Autodesk Inventor part; units mm, degrees
ref_plane "YZ Plane" through (0, 0, 0) normal (1, 0, 0) x (0, 1, 0)
ref_plane "XZ Plane" through (0, 0, 0) normal (0, 1, 0) x (-1, 0, 0)
ref_plane "Arbeitsebene1" through (0, 0, -6) normal (0, 0, 1) x (1, 0, 0)
sketch "Skizze1" plane through (0, 0, -6) normal (0, 0, 1) x (1, 0, 0)
  circle A0 centre (0, 42) radius 6
  circle A1 centre (50, 42) radius 6
  circle A2 centre (50, 0) radius 6
  circle A3 centre (0, 0) radius 6
  line L0 (6.489, 48.9995) -> (6.489, 49.9028)
  line L1 (6.489, 49.9028) -> (-6, 49.9028)
  line L2 (-6, 49.9028) -> (-6, -8.0972)
  line L3 (-6, -8.0972) -> (5.7305, -8.0972)
  line L4 (5.7305, -8.0972) -> (5.7305, -4.6433)
  line L5 (5.7305, -4.6433) -> (25.1643, -4.6433)
  line L6 (25.1643, -4.6433) -> (13.6183, -0.9927)
  line L7 (13.6183, -0.9927) -> (6.9629, 3.2)
  line L8 (6.9629, 3.2) -> (-0.5, 23.5649)
  line L9 (-0.5, 23.5649) -> (2.346, 34.9379)
  line L10 (2.346, 34.9379) -> (18.55, 40.876)
  line L11 (18.55, 40.876) -> (19.7446, 48.9995)
  line L12 (19.7446, 48.9995) -> (6.489, 48.9995)
  circle A4 centre (0, 42) radius 3.2
  circle A5 centre (0, 0) radius 3.2
  line L13 (-6, -8.0972) -> (56, -8.0972)
  line L14 (56, -8.0972) -> (56, 49.9028)
  line L15 (56, 49.9028) -> (-6, 49.9028)
  line L16 (-6, 49.9028) -> (-6, -8.0972)
  circle A6 centre (25, 19) radius 21
  line L17 (22.1022, 54.5009) -> (31.9971, 38.8) construction
  line L18 (31.9971, 54.5009) -> (22.1022, 38.8) construction
  point P0 (0, 0)
extrude "Extrusion1" add sketch "Skizze1" along normal blind 6 contours L2 L1 L0 L12 L11 L10 L9 L8 L7 L6 L5 L4 L3 | L15 L14 L13 L4 L5 L6 L7 L8 L9 L10 L11 L12 L0 | A6
sketch "Skizze2" plane through (0, 0, 0) normal (0, 0, 1) x (1, 0, 0)
  circle A0 centre (0, 42) radius 6
  circle A1 centre (0, 0) radius 6
  line L0 (56, -8.0972) -> (56, 0)
  circle A2 centre (50, 0) radius 6
  line L1 (56, 0) -> (56, 42)
  circle A3 centre (50, 42) radius 6
  line L2 (56, 42) -> (56, 49.9028)
  line L3 (56, 49.9028) -> (-6, 49.9028)
  line L4 (-6, 42) -> (-6, 0)
  circle A4 centre (-6, 21) radius 14
  line L5 (56, 0) -> (56, 42)
  circle A5 centre (56, 21) radius 14
  line L6 (-6, -8.0972) -> (56, -8.0972)
  circle A6 centre (25, -8.0972) radius 15
  line L7 (-6, -8.0972) -> (56, -8.0972)
  line L8 (-6, 49.9028) -> (-6, 42)
  line L9 (-6, 42) -> (-6, 0)
  line L10 (-6, 0) -> (-6, -8.0972)
  point P0 (0, 0)
  dimension "d3" = 28
  dimension "d4" = 28
  dimension "d5" = 30
extrude "Extrusion2" cut sketch "Skizze2" against normal blind 6 contours A4 L4 | L4 A4 | A5 L1 | L1 A5 | A6 L6 | L6 A6
fillet "Rundung1" radius 6 10 edges at (56, 35, -3) (56, 7, -3) (56, 49.9028, -3) (56, -8.0972, -3) (40, -8.0972, -3) (10, -8.0972, -3) (-6, -8.0972, -3) (-6, 7, -3) (-6, 35, -3) (-6, 49.9028, -3)
sketch "Skizze4" plane through (0, 0, 0) normal (0, 0, 1) x (1, 0, 0)
  arc A0 (0, 49.9028) -> (-6, 43.9028) centre (0, 43.9028) ccw
  line L0 (-6, 43.9028) -> (-6, 42)
  circle A1 centre (0, 42) radius 6
  line L1 (-6, 42) -> (-6, 40.0788)
  arc A2 (-6, 40.0788) -> (-1.8, 34.3551) centre (0, 40.0788) ccw
  arc A3 (-1.8, 7.6449) -> (-1.8, 34.3551) centre (-6, 21) ccw
  arc A4 (-1.8, 7.6449) -> (-6, 1.9212) centre (0, 1.9212) ccw
  line L2 (-6, 1.9212) -> (-6, 0)
  circle A5 centre (0, 0) radius 6
  line L3 (-6, 0) -> (-6, -2.0972)
  arc A6 (-6, -2.0972) -> (0, -8.0972) centre (0, -2.0972) ccw
  line L4 (0, -8.0972) -> (4.8754, -8.0972)
  arc A7 (4.8754, -8.0972) -> (10.6253, -3.8115) centre (4.8754, -2.0972) ccw
  arc A8 (39.3747, -3.8115) -> (10.6253, -3.8115) centre (25, -8.0972) ccw
  arc A9 (39.3747, -3.8115) -> (45.1246, -8.0972) centre (45.1246, -2.0972) ccw
  line L5 (45.1246, -8.0972) -> (50, -8.0972)
  arc A10 (50, -8.0972) -> (56, -2.0972) centre (50, -2.0972) ccw
  line L6 (56, -2.0972) -> (56, 0)
  circle A11 centre (50, 0) radius 6
  line L7 (56, 0) -> (56, 1.9212)
  arc A12 (56, 1.9212) -> (51.8, 7.6449) centre (50, 1.9212) ccw
  arc A13 (51.8, 34.3551) -> (51.8, 7.6449) centre (56, 21) ccw
  arc A14 (51.8, 34.3551) -> (56, 40.0788) centre (50, 40.0788) ccw
  line L8 (56, 40.0788) -> (56, 42)
  circle A15 centre (50, 42) radius 6
  line L9 (56, 42) -> (56, 43.9028)
  arc A16 (56, 43.9028) -> (50, 49.9028) centre (50, 43.9028) ccw
  line L10 (50, 49.9028) -> (0, 49.9028)
  line L11 (6.6, 89.7038) -> (6.6, 65.7038)
  line L12 (6.6, 65.7038) -> (31.6, 65.7038)
  line L13 (31.6, 65.7038) -> (31.6, 89.7038)
  line L14 (31.6, 89.7038) -> (6.6, 89.7038)
  circle A17 centre (29.6, 87.7038) radius 1.05
  circle A18 centre (29.6, 75.2038) radius 1.05
  circle A19 centre (8.6, 75.2038) radius 1.05
  circle A20 centre (8.6, 87.7038) radius 1.05
  line L15 (27.8, 85.1038) -> (26.58, 85.1038)
  line L16 (27.8, 84.3038) -> (27.8, 85.1038)
  line L17 (26.58, 84.3038) -> (27.8, 84.3038)
  line L18 (26.58, 85.1038) -> (26.58, 84.3038)
  line L19 (50, 49.9028) -> (0, 49.9028)
  line L20 (31.6, 49.9028) -> (6.6, 49.9028)
  line L21 (6.6, 49.9028) -> (6.6, 51.9028)
  line L22 (6.6, 51.9028) -> (31.6, 51.9028)
  line L23 (31.6, 51.9028) -> (31.6, 49.9028)
  point P0 (0, 0)
  dimension "d13" = 2
extrude "Extrusion4" add sketch "Skizze4" against normal blind 6 contours L21 L22 L23 L10
properties part number "20_Schlitten"
Read the model definition and answer for the solid it produces. Units are mm, in the model's axes. A direction names the side the tool comes from. Round coordinates to 2 decimals unless told otherwise and drop trailing zeros. Write each loop counter-clockwise with the first axis right and the second up, starting at its lowest first coordinate (ties: lowest second). Pieces come first, ordered by that corner, then holes.
1. The part is cut by section B-B, the plane x = 49. Determine the outline of the cut face in (y, z), then the cut area to 3 significant figures.
2. The part is cut by section D-D, the plane y = 30. Determine the outline of the cut face in (x, z).
3. Given pin 1 Ø7 at (x, y) = (50, 42) entering from -Z; pin 2 Ø2 at (y, z) = (17.5, -2.5) entering from +X; pin 3 Ø1.6 at (y, z) = (51, -2) entering from +X; pin 4 Ø2 at (y, z) = (51, -2.5) entering from -X, each flat-ended and moving along its own axis, determine where each tip first touches the part or whether it passes through.
4. Which of the six approach directions +Z, -Z, +X, -X, +Y, -Y give full straight-line access (tool end or side, diameter ignored) to faces 4 (the face through (41, 49.903, -3)), 5 (the face through (54.81, 36.49, -2.96)), 6 (the face through (8.42, -6.94, -2.96))?
5. Straight lines are drawn through the part: L1, parallel to X at y = 2.5, z = -1; L2, parallel to Y at x = -1, z = -2.8; L3, parallel to Y at x = 50, z = -2. For each, find the intervals that lie inside material, in ascending order.
6. The part is cut by section C-C, the plane y = 4. Determine the outline of the cut face in (x, z).
7. Determine the mould class of faces 1 (the face through (19, 51.903, -3)), 2 (the face through (-6, 40.6, -3)), 3 (the face through (54.869, 5.428, -2.958)) for opening direction Y: pulls with the +Y half, pulls with the -Y half, needs draft (parallel to the pull), parting line crosses it, or undercut.
Values:
1. outline: (-8.1, -6) - (-5.92, -6) - (-5.92, 0) - (-8.1, 0) - close; (5.92, -6) - (8.88, -6) - (8.88, 0) - (5.92, 0) - close; (33.12, -6) - (36.08, -6) - (36.08, 0) - (33.12, 0) - close; (47.92, -6) - (49.9, -6) - (49.9, 0) - (47.92, 0) - close
1. area: 60.5 mm2
2. outline: (4.72, -6) - (45.28, -6) - (45.28, 0) - (4.72, 0) - close
3. pin 1: passes through
3. pin 2: stops at x = 42.74
3. pin 3: stops at x = 31.6
3. pin 4: stops at x = 6.6
4. face 4: +Z, -Z, +X, +Y
4. face 5: +Z, -Z, +X
4. face 6: +Z, -Z, -Y
5. L1: x = -5.97 to -5.45, 5.45 to 14.38, 35.62 to 44.55, 55.45 to 55.97
5. L2: y = -8.01 to -5.92, 5.92 to 7.92, 34.08 to 36.08, 47.92 to 49.82
5. L3: y = -8.1 to -6, 6 to 8.35, 33.65 to 36, 48 to 49.9
6. outline: (-5.63, -6) - (-4.47, -6) - (-4.47, 0) - (-5.63, 0) - close; (4.47, -6) - (16.13, -6) - (16.13, 0) - (4.47, 0) - close; (33.87, -6) - (45.53, -6) - (45.53, 0) - (33.87, 0) - close; (54.47, -6) - (55.63, -6) - (55.63, 0) - (54.47, 0) - close
7. face 1: pulls with the +Y half
7. face 2: needs draft
7. face 3: undercut
